from build123d import *

# Parameters (mm, degrees)
F2_SIZE  = 5.08
F3_SIZE  = 5.08
F4_R     = 18.147419
F5_DEPTH = 127.908953


with BuildPart() as f1:
    # F0 (on Front) → F1 (revolve)
    with BuildSketch(Plane.XZ):
        Polygon((0, 51.78383), (0, 86.945966), (-23.790576, 86.945966), (-23.790576, 0), (0, 0), (104.118377, 0), (104.118377, 20.117693), (82.508355, 20.117693), (82.508355, 35.376113), (50.429285, 35.376113), (50.429285, 51.78383), align=None)
    revolve(axis=Axis((-54.851383, 0, 0), (1, 0, 0)))

    # F2
    f2_edges = [f1.edges().sort_by_distance(p)[0] for p in [
        (0, 0, -51.78383),
    ]]
    chamfer(f2_edges, length=F2_SIZE)

    # F3
    f3_edges = [f1.edges().sort_by_distance(p)[0] for p in [
        (50.429285, 0, -35.376113),
        (82.508355, 0, -20.117693),
    ]]
    chamfer(f3_edges, length=F3_SIZE)

    # F4 (on face) → F5 (cut, through all)
    with BuildSketch(Plane(origin=(-23.790576, 0, 0), x_dir=(0, -1, 0), z_dir=(-1, 0, 0))):
        Circle(F4_R)
    extrude(amount=-F5_DEPTH, mode=Mode.SUBTRACT)


solid = f1.part
The model under review builds one solid part; all positions refer to its coordinate system, in mm. A direction names the side the tool comes from. Coordinates: 2 decimals unless noted, no trailing zeros. Write each loop counter-clockwise with the first axis right and the second up, starting at its lowest first coordinate (ties: lowest second). Pieces come first, ordered by that corner, then holes. Notation, with made-up numbers: (65.5, -20) - (109.5, -20) arc R31 cw to (109.5, 14) - close; hole circle Ø1 at (54, 31.25). An arc over 180 degrees is marked (long way). Answer as a JSON object with one key per item and string values. Group by question number.
1. Machinability: for faces 4 (the face through (82.508, -24.1, 8.4)), 5 (the face through (-12.06, -26.12, 82.93)), which of the approach directions +Z, -Z, +X, -X, +Y, -Y give a long, thin tool a straight path to every point of the face, cutting with its end or side? Answer none if there is none.
2. Add section D-D (x = 95.5). Give the boundary of the cut face in (y, z).
3. Clearance check with flat-ended pins moving along their axes: pin 1 Ø10 at (y, z) = (-65, -28.5) entering from +X; pin 2 Ø1 at (y, z) = (-35.5, 34) entering from +X; pin 3 Ø2 at (y, z) = (-1, -31.5) entering from +X. State where each tip first meets the part, or that it passes through.
4. Mouldability with a two-part tool opening along Z and no side actions: class faces 1 (the face through (104.118, -15, 11)), 2 (the face through (39.269, 3.934, -17.716)), 3 (the face through (95.74, 19.64, -4.36)) as pulls with the +Z half, pulls with the -Z half, needs draft (parallel to the pull), parting line crosses it, or undercut.
5. Add section C-C (x = -13). Give the boundary of the cut face in (y, z).
6. To check wall thickness, follow probe 1 along Z at (x, y) = (39, 0); probe 2 along Z at (x, y) = (76.5, 0); probe 3 along Y at (x, z) = (-15.5, -12). State the ranges of each line that lie inside material, in increasing order.
7. Add section A-A (y = 0). Give the boundary of the cut face in (x, z).
Findings:
{
 "1": {"face 4": "+X", "face 5": "+X, -X"},
 "2": {"outline": "circle Ø40.24 at (0, 0); hole circle Ø36.29 at (0, 0)"},
 "3": {"pin 1": "x = 0", "pin 2": "x = 50.43", "pin 3": "x = 82.51"},
 "4": {"face 1": "needs draft", "face 2": "undercut", "face 3": "parting line crosses it"},
 "5": {"outline": "circle Ø173.89 at (0, 0); hole circle Ø36.29 at (0, 0)"},
 "6": {"probe 1": "-51.78 to -18.15, 18.15 to 51.78", "probe 2": "-35.38 to -18.15, 18.15 to 35.38", "probe 3": "-86.11 to -13.61, 13.61 to 86.11"},
 "7": {"outline": "(-23.79, -86.95) - (0, -86.95) - (0, -56.86) - (5.08, -51.78) - (50.43, -51.78) - (50.43, -40.46) - (55.51, -35.38) - (82.51, -35.38) - (82.51, -25.2) - (87.59, -20.12) - (104.12, -20.12) - (104.12, -18.15) - (-23.79, -18.15) - close; (-23.79, 18.15) - (104.12, 18.15) - (104.12, 20.12) - (87.59, 20.12) - (82.51, 25.2) - (82.51, 35.38) - (55.51, 35.38) - (50.43, 40.46) - (50.43, 51.78) - (5.08, 51.78) - (0, 56.86) - (0, 86.95) - (-23.79, 86.95) - close"}
}
